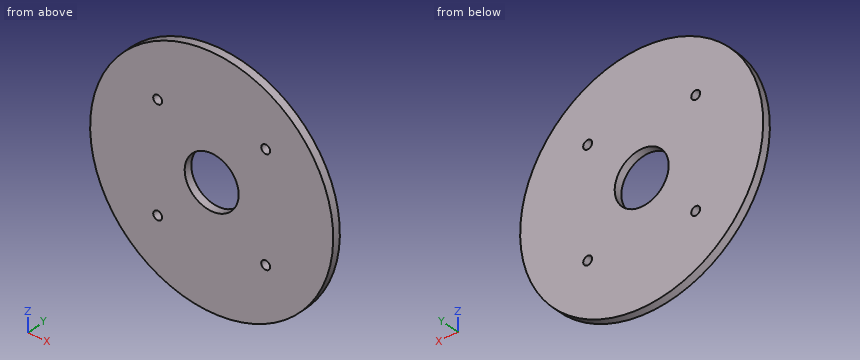
```python
from build123d import *

# Parameters (mm, degrees)
SKETCH1_R           = 45
SKETCH1_R_2         = 10
BOSS_EXTRUDE1_DEPTH = 1.5
SKETCH2_R           = 1.65
CUT_EXTRUDE1_DEPTH  = 10


with BuildPart() as part:
    # Sketch1 → Boss-Extrude1 (new, symmetric)
    with BuildSketch(Plane(origin=(0, 0, 0), x_dir=(1, 0, 0), z_dir=(0, 1, 0))):
        with Locations(Location((0, 0, 0), (0, 0, 270))):
            Circle(SKETCH1_R)
        with Locations(Location((0, 0, 0), (0, 0, 270))):
            Circle(SKETCH1_R_2, mode=Mode.SUBTRACT)
    extrude(amount=BOSS_EXTRUDE1_DEPTH, both=True)

    # Sketch2 → Cut-Extrude1 (cut)
    with BuildSketch(Plane(origin=(0, 1.5, 0), x_dir=(1, 0, 0), z_dir=(0, 1, 0))):
        with Locations(Location((-20, -20, 0), (0, 0, 270))):
            Circle(SKETCH2_R)
        with Locations(Location((-20, 20, 0), (0, 0, 270))):
            Circle(SKETCH2_R)
        with Locations(Location((20, 20, 0), (0, 0, 270))):
            Circle(SKETCH2_R)
        with Locations(Location((20, -20, 0), (0, 0, 270))):
            Circle(SKETCH2_R)
    extrude(amount=-CUT_EXTRUDE1_DEPTH, mode=Mode.SUBTRACT)


solid = part.part
```
Geometry: final body of the model. Coordinates: model frame, mm. Round coordinates to 2 decimals unless told otherwise and drop trailing zeros. Write each loop counter-clockwise with the first axis right and the second up, starting at its lowest first coordinate (ties: lowest second). Pieces come first, ordered by that corner, then holes.
Item 1: Section query A-A (z = 0). Return loops of the section in (x, y), plus the area to 3 significant figures.
Item 2: Section query D-D (x = -20). Return loops of the section in (y, z).
Item 3: Section query B-B (x = 0). Return loops of the section in (y, z).
Item 4: Section query C-C (y = -0.05). Return loops of the section in (x, z), plus the area to 3 significant figures.
Item 5: Material intervals for L1, parallel to X at y = -0.85, z = -20; L2, parallel to X at y = -1.25, z = 7.5; L3, parallel to X at y = 0.75, z = 3, sorted ascending.
Completed:
1. outline: (-45, -1.5) - (-10, -1.5) - (-10, 1.5) - (-45, 1.5) - close; (10, -1.5) - (45, -1.5) - (45, 1.5) - (10, 1.5) - close
1. area: 210 mm2
2. outline: (-1.5, -40.31) - (1.5, -40.31) - (1.5, -21.65) - (-1.5, -21.65) - close; (-1.5, -18.35) - (1.5, -18.35) - (1.5, 18.35) - (-1.5, 18.35) - close; (-1.5, 21.65) - (1.5, 21.65) - (1.5, 40.31) - (-1.5, 40.31) - close
3. outline: (-1.5, -45) - (1.5, -45) - (1.5, -10) - (-1.5, -10) - close; (-1.5, 10) - (1.5, 10) - (1.5, 45) - (-1.5, 45) - close
4. outline: circle Ø90 at (0, 0); hole circle Ø3.3 at (-20, -20); hole circle Ø3.3 at (-20, 20); hole circle Ø20 at (0, 0); hole circle Ø3.3 at (20, -20); hole circle Ø3.3 at (20, 20)
4. area: 6,010 mm2
5. L1: x = -40.31 to -21.65, -18.35 to 18.35, 21.65 to 40.31
5. L2: x = -44.37 to -6.61, 6.61 to 44.37
5. L3: x = -44.9 to -9.54, 9.54 to 44.9
